Verification items for the finished model (mm, model axes). Face numbers are marked on the shaded views. Coordinates: 2 decimals unless noted, no trailing zeros. Order: outer loops, then holes, each group sorted by start corner. A loop starts at its lowest first (then second) coordinate and runs counter-clockwise, first axis right, second up. Notation, with made-up numbers: (11, 8) -> (70, 8) arc R22 ccw to (70, 36) -> close; hole circle Ø9 at (-39.5, 50.5). An arc over 180 degrees is marked (long way). Use CSV: the item, a comma, the result in double quotes. Start each with the question number.
1) Scan lines: line 1 along Z through (x, y) = (2, 0); line 2 along Y through (x, z) = (1.45, -0.75); line 3 along Z through (x, y) = (2.3, -1.75). Record each from-to range of solid material in increasing order.
2) Sectioned sample at C-C on x = 2.8. Record the boundary of the cut face in (y, z), then the cut area to 3 significant figures.
3) Release check for a two-part mould opening along Z. For the marked faces 1 and 2 record: released by +Z, released by -Z, zero draft, split by the parting line, or undercut.
4) Sectioned sample at A-A on y = 0. Record the boundary of the cut face in (x, z), then the cut area to 3 significant figures.
5) Go/stop test with a flat-tipped pin: pin 1 (3.5 mm diameter, centred on y = 0, z = 0, fed in from +X). Record where the tip stops, or that it passes through.
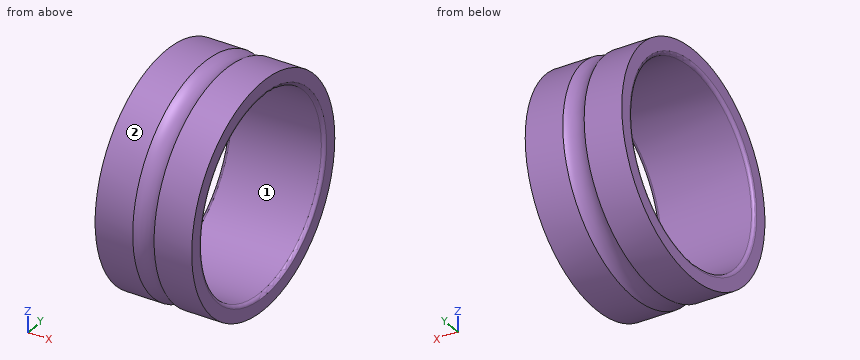
Autodesk Inventor part; units mm, degrees
ref_plane "ip_st_1_1_XY" through (1.5, 4, 0) normal (1, 0, 0) x (0, 0, -1)
ref_plane "ip_st_1_1_YZ" through (1.5, 4, 0) normal (0, 0, -1) x (0, 1, 0)
ref_plane "ip_st_1_1_ZX" through (1.5, 4, 0) normal (0, 1, 0) x (1, 0, 0)
sketch "Sketch_1" plane through (0, 0, 0) normal (0, 0, 1) x (1, 0, 0)
  line L0 (3, 0) -> (0, 0)
  arc A0 (0, 3.1) -> (0.1, 3) centre (0.1, 3.1) ccw
  line L1 (0.1, 3) -> (2.9, 3)
  arc A1 (2.9, 3) -> (3, 3.1) centre (2.9, 3.1) ccw
  line L2 (3, 3.1) -> (3, 3.5)
  line L3 (3, 3.5) -> (1.8317, 3.5)
  arc A2 (1.1683, 3.5) -> (1.8317, 3.5) centre (1.5, 4) ccw
  line L4 (1.1683, 3.5) -> (0, 3.5)
  line L5 (0, 3.5) -> (0, 3.1)
revolve "Revolution1" add sketch "Sketch_1" angle 360 about axis through (3, 0, 0) along (1, 0, 0)
ref_plane "ip_st_1_1_XY" through (1.5, 4, 0) normal (1, 0, 0) x (0, 0, -1)
ref_plane "ip_st_1_1_YZ" through (1.5, 4, 0) normal (0, 0, -1) x (0, 1, 0)
ref_plane "ip_st_1_1_ZX" through (1.5, 4, 0) normal (0, 1, 0) x (1, 0, 0)
ref_plane "ip_st_1_10_XY" through (1.5, -3.6955, -1.5307) normal (1, 0, 0) x (0, 0, -1)
ref_plane "ip_st_1_10_YZ" through (1.5, -3.6955, -1.5307) normal (0, 0, -1) x (0, 1, 0)
ref_plane "ip_st_1_10_ZX" through (1.5, -3.6955, -1.5307) normal (0, 1, 0) x (1, 0, 0)
ref_plane "ip_st_1_11_XY" through (1.5, -2.8284, -2.8284) normal (1, 0, 0) x (0, 0, -1)
ref_plane "ip_st_1_11_YZ" through (1.5, -2.8284, -2.8284) normal (0, 0, -1) x (0, 1, 0)
ref_plane "ip_st_1_11_ZX" through (1.5, -2.8284, -2.8284) normal (0, 1, 0) x (1, 0, 0)
ref_plane "ip_st_1_12_XY" through (1.5, -1.5307, -3.6955) normal (1, 0, 0) x (0, 0, -1)
ref_plane "ip_st_1_12_YZ" through (1.5, -1.5307, -3.6955) normal (0, 0, -1) x (0, 1, 0)
ref_plane "ip_st_1_12_ZX" through (1.5, -1.5307, -3.6955) normal (0, 1, 0) x (1, 0, 0)
ref_plane "ip_st_1_13_XY" through (1.5, 0, -4) normal (1, 0, 0) x (0, 0, -1)
ref_plane "ip_st_1_13_YZ" through (1.5, 0, -4) normal (0, 0, -1) x (0, 1, 0)
ref_plane "ip_st_1_13_ZX" through (1.5, 0, -4) normal (0, 1, 0) x (1, 0, 0)
ref_plane "ip_st_1_14_XY" through (1.5, 1.5307, -3.6955) normal (1, 0, 0) x (0, 0, -1)
ref_plane "ip_st_1_14_YZ" through (1.5, 1.5307, -3.6955) normal (0, 0, -1) x (0, 1, 0)
ref_plane "ip_st_1_14_ZX" through (1.5, 1.5307, -3.6955) normal (0, 1, 0) x (1, 0, 0)
ref_plane "ip_st_1_15_XY" through (1.5, 2.8284, -2.8284) normal (1, 0, 0) x (0, 0, -1)
ref_plane "ip_st_1_15_YZ" through (1.5, 2.8284, -2.8284) normal (0, 0, -1) x (0, 1, 0)
ref_plane "ip_st_1_15_ZX" through (1.5, 2.8284, -2.8284) normal (0, 1, 0) x (1, 0, 0)
ref_plane "ip_st_1_16_XY" through (1.5, 3.6955, -1.5307) normal (1, 0, 0) x (0, 0, -1)
ref_plane "ip_st_1_16_YZ" through (1.5, 3.6955, -1.5307) normal (0, 0, -1) x (0, 1, 0)
ref_plane "ip_st_1_16_ZX" through (1.5, 3.6955, -1.5307) normal (0, 1, 0) x (1, 0, 0)
ref_plane "ip_st_1_2_XY" through (1.5, 3.6955, 1.5307) normal (1, 0, 0) x (0, 0, -1)
ref_plane "ip_st_1_2_YZ" through (1.5, 3.6955, 1.5307) normal (0, 0, -1) x (0, 1, 0)
ref_plane "ip_st_1_2_ZX" through (1.5, 3.6955, 1.5307) normal (0, 1, 0) x (1, 0, 0)
ref_plane "ip_st_1_3_XY" through (1.5, 2.8284, 2.8284) normal (1, 0, 0) x (0, 0, -1)
ref_plane "ip_st_1_3_YZ" through (1.5, 2.8284, 2.8284) normal (0, 0, -1) x (0, 1, 0)
ref_plane "ip_st_1_3_ZX" through (1.5, 2.8284, 2.8284) normal (0, 1, 0) x (1, 0, 0)
ref_plane "ip_st_1_4_XY" through (1.5, 1.5307, 3.6955) normal (1, 0, 0) x (0, 0, -1)
ref_plane "ip_st_1_4_YZ" through (1.5, 1.5307, 3.6955) normal (0, 0, -1) x (0, 1, 0)
ref_plane "ip_st_1_4_ZX" through (1.5, 1.5307, 3.6955) normal (0, 1, 0) x (1, 0, 0)
ref_plane "ip_st_1_5_XY" through (1.5, 0, 4) normal (1, 0, 0) x (0, 0, -1)
ref_plane "ip_st_1_5_YZ" through (1.5, 0, 4) normal (0, 0, -1) x (0, 1, 0)
ref_plane "ip_st_1_5_ZX" through (1.5, 0, 4) normal (0, 1, 0) x (1, 0, 0)
ref_plane "ip_st_1_6_XY" through (1.5, -1.5307, 3.6955) normal (1, 0, 0) x (0, 0, -1)
ref_plane "ip_st_1_6_YZ" through (1.5, -1.5307, 3.6955) normal (0, 0, -1) x (0, 1, 0)
ref_plane "ip_st_1_6_ZX" through (1.5, -1.5307, 3.6955) normal (0, 1, 0) x (1, 0, 0)
ref_plane "ip_st_1_7_XY" through (1.5, -2.8284, 2.8284) normal (1, 0, 0) x (0, 0, -1)
ref_plane "ip_st_1_7_YZ" through (1.5, -2.8284, 2.8284) normal (0, 0, -1) x (0, 1, 0)
ref_plane "ip_st_1_7_ZX" through (1.5, -2.8284, 2.8284) normal (0, 1, 0) x (1, 0, 0)
ref_plane "ip_st_1_8_XY" through (1.5, -3.6955, 1.5307) normal (1, 0, 0) x (0, 0, -1)
ref_plane "ip_st_1_8_YZ" through (1.5, -3.6955, 1.5307) normal (0, 0, -1) x (0, 1, 0)
ref_plane "ip_st_1_8_ZX" through (1.5, -3.6955, 1.5307) normal (0, 1, 0) x (1, 0, 0)
ref_plane "ip_st_1_9_XY" through (1.5, -4, 0) normal (1, 0, 0) x (0, 0, -1)
ref_plane "ip_st_1_9_YZ" through (1.5, -4, 0) normal (0, 0, -1) x (0, 1, 0)
ref_plane "ip_st_1_9_ZX" through (1.5, -4, 0) normal (0, 1, 0) x (1, 0, 0)
ref_plane "ip_st_1a_XY" through (0, 0, 0) normal (1, 0, 0) x (0, 0, -1)
ref_plane "ip_st_1a_YZ" through (0, 0, 0) normal (0, 0, -1) x (0, 1, 0)
ref_plane "ip_st_1a_ZX" through (0, 0, 0) normal (0, 1, 0) x (1, 0, 0)
ref_plane "ip_st_2a_XY" through (0.1875, 0, 0) normal (1, 0, 0) x (0, 0, -1)
ref_plane "ip_st_2a_YZ" through (0.1875, 0, 0) normal (0, 0, -1) x (0, 1, 0)
ref_plane "ip_st_2a_ZX" through (0.1875, 0, 0) normal (0, 1, 0) x (1, 0, 0)
properties part number "MF106ZZ1 Inner Ring"
Answers follow:
1,line 1,"z = -3.5 to -3, 3 to 3.5"
1,line 2,"y = -3.32 to -2.9, 2.9 to 3.32"
1,line 3,"z = -3.03 to -2.44, 2.44 to 3.03"
2,outline,"circle Ø7 at (0, 0); hole circle Ø6 at (0, 0)"
2,area,"10.2 mm²"
3,face 1,"undercut"
3,face 2,"split by the parting line"
4,outline,"(0, -3.5) -> (1.17, -3.5) arc R0.6 cw to (1.83, -3.5) -> (3, -3.5) -> (3, -3.1) arc R0.1 ccw to (2.9, -3) -> (0.1, -3) arc R0.1 ccw to (0, -3.1) -> close; (0, 3.1) arc R0.1 ccw to (0.1, 3) -> (2.9, 3) arc R0.1 ccw to (3, 3.1) -> (3, 3.5) -> (1.83, 3.5) arc R0.6 cw to (1.17, 3.5) -> (0, 3.5) -> close"
4,area,"2.90 mm²"
5,pin 1,"passes through"
